Geometry check sheet. Reference: the model listing, model coordinates, mm. A direction names the side the tool comes from. Coordinates: 2 decimals unless noted, no trailing zeros. Write each loop counter-clockwise with the first axis right and the second up, starting at its lowest first coordinate (ties: lowest second). Pieces come first, ordered by that corner, then holes.
from build123d import *

# Parameters (mm, degrees)
F0_R     = 20
F0_R_2   = 7.5
F0_R_3   = 5
F1_DEPTH = 8
F2_DEPTH = 13
F3_R     = 2


with BuildPart() as f1:
    # F0 (on Front) → F1 (new body)
    with BuildSketch(Plane.XZ):
        Circle(F0_R)
        Circle(F0_R_2, mode=Mode.SUBTRACT)
        Circle(F0_R_2)
        Circle(F0_R_3, mode=Mode.SUBTRACT)
    extrude(amount=F1_DEPTH)

    # F0 (on Front) → F2 (join)
    with BuildSketch(Plane.XZ):
        Circle(F0_R_2)
        Circle(F0_R_3, mode=Mode.SUBTRACT)
    extrude(amount=F2_DEPTH)

    # F3
    f3_edges = [f1.edges().sort_by_distance(p)[0] for p in [
        (-20, 0, 0),
        (-20, -8, 0),
    ]]
    fillet(f3_edges, radius=F3_R)


solid = f1.part
1. Gauge pin test, flat ends, axial feed: pin 1 Ø6 at (x, z) = (0, 0) entering from +Y (3 decimals); pin 2 Ø2 at (x, y) = (0.5, -2) entering from -Z; pin 3 Ø4 at (y, z) = (-4, -13.5) entering from -X; pin 4 Ø3 at (x, y) = (-9.5, -5) entering from -Z. Record the tip position at first contact, or that the pin passes through.
Computed values:
pin 1: passes through
pin 2: stops at z = -20
pin 3: stops at x = -16.36
pin 4: stops at z = -18.33
2. Thickness scan on line 1 along Z through (x, y) = (0, -4); line 2 along Z through (x, y) = (0, -7.5); line 3 along Y through (x, z) = (-8.5, -16). Record the ranges inside material, lowest first.
Computed values:
line 1: z = -20 to -5, 5 to 20
line 2: z = -19.32 to -5, 5 to 19.32
line 3: y = -8 to 0
3. Sectioned sample at C-C, the plane y = -12. Record the boundary of the cut face in (x, z).
Computed values:
outline: circle Ø15 at (0, 0); hole circle Ø10 at (0, 0)
4. Access from +Z, -Z, +X, -X, +Y, -Y to the whole of each face (thin tool, end or side, straight path). Record for faces 4 (the cylindrical face through (-7.493, -10.465, 0.33)), 5 (the flat face through (4, 0, -4)).
Computed values:
face 4: -Y
face 5: +Z, -Z, +X, -X, +Y
5. Sectioned sample at B-B, the plane x = 0. Record the boundary of the cut face in (y, z).
Computed values:
outline: (-13, -7.5) - (-8, -7.5) - (-8, -18) arc R2 ccw to (-6, -20) - (-2, -20) arc R2 ccw to (0, -18) - (0, -5) - (-13, -5) - close; (-13, 5) - (0, 5) - (0, 18) arc R2 ccw to (-2, 20) - (-6, 20) arc R2 ccw to (-8, 18) - (-8, 7.5) - (-13, 7.5) - close
6. Sectioned sample at A-A, the plane z = 0. Record the boundary of the cut face in (x, y).
Computed values:
outline: (-20, -6) arc R2 ccw to (-18, -8) - (-7.5, -8) - (-7.5, -13) - (-5, -13) - (-5, 0) - (-18, 0) arc R2 ccw to (-20, -2) - close; (5, -13) - (7.5, -13) - (7.5, -8) - (18, -8) arc R2 ccw to (20, -6) - (20, -2) arc R2 ccw to (18, 0) - (5, 0) - close
7. Draft check along Z on faces 1 (the flat face through (0, -8, -8)), 2 (the cylindrical face through (-1.08, -6.41, -4.88)), 3 (the cylindrical face through (-4.336, -3.972, -19.524)). Enter one of: released by +Z, released by -Z, zero draft, split by the parting line, or undercut.
Computed values:
face 1: zero draft
face 2: undercut
face 3: split by the parting line
